The model under review builds one solid part; all positions refer to its coordinate system, in mm. Face numbers are marked on the shaded views. A direction names the side the tool comes from. Round coordinates to 2 decimals unless told otherwise and drop trailing zeros. Loops run counter-clockwise (first coordinate to the right, second up) from the corner with the lowest first, then second, coordinate; pieces in that order, holes last. Notation, with made-up numbers: (43, -12.75) - (101, -12.75) arc R32 cw to (101, 16.25) - close; hole circle Ø6 at (51.25, 53.25). An arc over 180 degrees is marked (long way). Answer as CSV lines item,"result".
from build123d import *

# Parameters (mm, degrees)
F0_R     = 6.25
F1_DEPTH = 3.5
F2_R     = 4.75
F3_DEPTH = 6.5
F4_R     = 4.7
F5_DEPTH = 22
F6_SIZE  = 0.5


with BuildPart() as f1:
    # F0 (on Front) → F1 (new body)
    with BuildSketch(Plane.XZ):
        Circle(F0_R)
    extrude(amount=-F1_DEPTH)

    # F2 (on face) → F3 (join)
    with BuildSketch(Plane(origin=(0, 3.5, 0), x_dir=(-1, 0, 0), z_dir=(0, 1, 0))):
        Circle(F2_R)
    extrude(amount=F3_DEPTH)

    # F4 (on face) → F5 (join)
    with BuildSketch(Plane(origin=(0, 10, 0), x_dir=(-1, 0, 0), z_dir=(0, 1, 0))):
        Circle(F4_R)
    extrude(amount=F5_DEPTH)

    # F6
    f6_edges = [f1.edges().sort_by_distance(p)[0] for p in [
        (4.7, 32, 0),
    ]]
    chamfer(f6_edges, length=F6_SIZE)


solid = f1.part
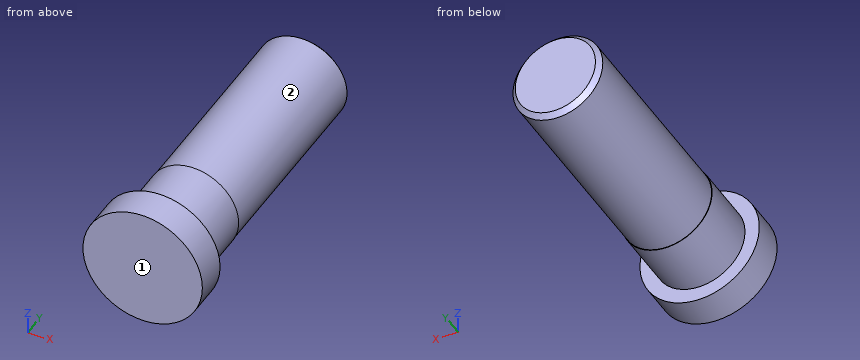
1. Clearance check with flat-ended pins moving along their axes: pin 1 (2 mm diameter, centred on x = 5, y = 18.5, fed in from -Z); pin 2 (6 mm diameter, centred on x = 5, y = 10.5, fed in from -Z); pin 3 (6 mm diameter, centred on x = 4.5, y = 27.5, fed in from -Z). State where each tip first meets the part, or that it passes through.
Numbers:
pin 1,"stops at z = -2.47"
pin 2,"stops at z = -4.29"
pin 3,"stops at z = -4.45"
2. Wall thickness on probe 1 along Y at (x, z) = (-2.5, 4.75); probe 2 along Z at (x, y) = (2, 4); probe 3 along X at (y, z) = (19.5, -2.75): over which ranges is each line inside the solid? List them lowest first.
Numbers:
probe 1,"y = 0 to 3.5"
probe 2,"z = -4.31 to 4.31"
probe 3,"x = -3.81 to 3.81"
3. Tool access review of the marked faces 1 and 2: name each direction out of +Z, -Z, +X, -X, +Y, -Y from which nothing blocks a thin tool from reaching the whole face with its end or side.
Numbers:
face 1,"+Z, -Z, +X, -X, -Y"
face 2,"+Y"
4. Take a section at C-C (y = 7). State the section outline as (x, z) points.
Numbers:
outline,"circle Ø9.5 at (0, 0)"
5. Take a section at D-D (y = 30.5). State the section outline as (x, z) points.
Numbers:
outline,"circle Ø9.4 at (0, 0)"
6. Take a section at A-A (z = 0). State the section outline as (x, y) points, plus the area to 3 significant figures.
Numbers:
outline,"(-6.25, 0) - (6.25, 0) - (6.25, 3.5) - (4.75, 3.5) - (4.75, 10) - (4.7, 10) - (4.7, 31.5) - (4.2, 32) - (-4.2, 32) - (-4.7, 31.5) - (-4.7, 10) - (-4.75, 10) - (-4.75, 3.5) - (-6.25, 3.5) - close"
area,"312 mm²"
7. Take a section at B-B (x = 0). State the section outline as (y, z) points.
Numbers:
outline,"(0, -6.25) - (3.5, -6.25) - (3.5, -4.75) - (10, -4.75) - (10, -4.7) - (31.5, -4.7) - (32, -4.2) - (32, 4.2) - (31.5, 4.7) - (10, 4.7) - (10, 4.75) - (3.5, 4.75) - (3.5, 6.25) - (0, 6.25) - close"
